Design review of the part built by this model. Coordinates are the model's own, in mm. Face numbers are marked on the shaded views. Give positions to 0.01 mm unless a question says otherwise; leave off trailing zeros. Write each loop counter-clockwise with the first axis right and the second up, starting at its lowest first coordinate (ties: lowest second). Pieces come first, ordered by that corner, then holes. Notation, with made-up numbers: M 25,63 L 74,63 A28 ccw 74,98 Z; hole C 70,17 d8. An arc over 180 degrees is marked long. Use one line per item in the form item = value. Start each with the question number.
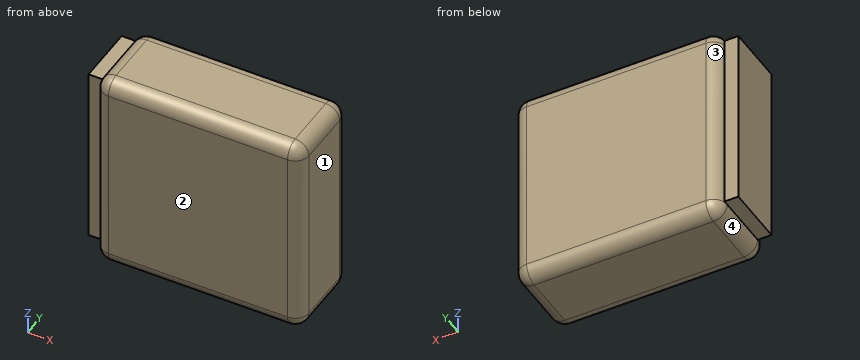
from build123d import *

# Parameters (mm, degrees)
SKETCH1_W           = 15
SKETCH1_H           = 15
BOSS_EXTRUDE1_DEPTH = 6
FILLET1_R           = 1
SKETCH2_W           = 13.272032768
SKETCH2_H           = 4.346157801
BOSS_EXTRUDE2_DEPTH = 1


with BuildPart() as part:
    # Sketch1 → Boss-Extrude1 (new body)
    with BuildSketch(Plane(origin=(0, 0, 0), x_dir=(1, 0, 0), z_dir=(0, 1, 0))):
        with Locations((-12.287002789, -4.651800626)):
            Rectangle(SKETCH1_W, SKETCH1_H)
    extrude(amount=BOSS_EXTRUDE1_DEPTH)

    # Fillet1
    fillet1_edges = [part.edges().sort_by_distance(p)[0] for p in [
        (-4.787002789, 6, 4.651800626),
        (-12.287002789, 6, -2.848199374),
        (-19.787002789, 6, 4.651800626),
        (-12.287002789, 0, -2.848199374),
        (-4.787002789, 0, 4.651800626),
        (-12.287002789, 0, 12.151800626),
        (-19.787002789, 0, 4.651800626),
        (-12.287002789, 6, 12.151800626),
        (-19.787002789, 3, -2.848199374),
        (-4.787002789, 3, -2.848199374),
        (-4.787002789, 3, 12.151800626),
        (-19.787002789, 3, 12.151800626),
    ]]
    fillet(fillet1_edges, radius=FILLET1_R)

    # Sketch2 → Boss-Extrude2 (add)
    with BuildSketch(Plane.ZY.offset(19.787002789)):
        with Locations((4.78781701, 3.173078901)):
            Rectangle(SKETCH2_W, SKETCH2_H)
    extrude(amount=BOSS_EXTRUDE2_DEPTH)


solid = part.part
1. Clearance check with flat-ended pins moving along their axes: pin 1 Ø0.8 at (x, z) = (-20, 3.5) entering from -Y; pin 2 Ø3 at (x, y) = (-19, 1.5) entering from +Z; pin 3 Ø1.1 at (x, y) = (-20, 3.5) entering from +Z; pin 4 Ø0.8 at (x, z) = (-20, 4.5) entering from +Y. State where each tip first meets the part, or that it passes through.
2. To check wall thickness, follow L1, parallel to X at y = 0.95, z = 3.25; L2, parallel to X at y = 5.65, z = 11; L3, parallel to Z at x = -19.5, y = 2.1. State the ranges of each line that lie inside material, in increasing order.
3. Draft analysis for pull direction X (two halves, no side actions). For the marked faces 1, 2, 3 and 4, state which applies: pulls with the +X half, pulls with the -X half, needs draft (parallel to the pull), parting line crosses it, or undercut.
4. We need section A-A (z = 0.5). State the section outline as (x, y) points, and give its area (3 significant figures).
5. We need section B-B (x = -19.5). State the section outline as (y, z) points, and give its area (3 significant figures).
Answer block:
q1.pin_1 = 0.42
q1.pin_2 = 12.15
q1.pin_3 = 11.9
q1.pin_4 = 5.58
q2.L1 = -19.79 to -4.79
q2.L2 = -19.55 to -5.03
q2.L3 = -2.55 to 11.85
q3.face_1 = pulls with the +X half
q3.face_2 = needs draft
q3.face_3 = undercut
q3.face_4 = pulls with the -X half
q4.outline = M -20.79,1 L -19.79,1 A1 ccw -18.79,0 L -5.79,0 A1 ccw -4.79,1 L -4.79,5 A1 ccw -5.79,6 L -18.79,6 A1 ccw -19.79,5 L -19.79,5.35 L -20.79,5.35 Z
q4.area = 93.5 mm^2
q5.outline = M 0.3,-1.85 A0.7 ccw 1,-2.55 L 5,-2.55 A0.7 ccw 5.7,-1.85 L 5.7,11.15 A0.7 ccw 5,11.85 L 1,11.85 A0.7 ccw 0.3,11.15 Z
q5.area = 77.4 mm^2
